Solid Edge part; units mm, degrees
sketch "Sketch1" plane through (0, 0, 0) normal (0, 0, 1) x (1, 0, 0)
  line L0 (0, 0) -> (70, 0)
  line L1 (70, 0) -> (70, 50)
  line L2 (70, 50) -> (0, 50)
  line L3 (0, 50) -> (0, 0)
extrude "Protrusion1" add sketch "Sketch1" along normal blind 5
sketch "Sketch2" plane through (0, 0, 0) normal (0, 0, 1) x (1, 0, 0)
  line L0 (25, 12.5) -> (25, 37.5)
  line L1 (25, 37.5) -> (20, 37.5)
  line L2 (20, 37.5) -> (20, 12.5)
  line L3 (20, 12.5) -> (25, 12.5)
extrude "ExtrudedProtrusion_2" add sketch "Sketch2" against normal blind 30
sketch "Sketch3" plane through (25, 25, -6.7078) normal (1, 0, 0) x (0, -1, 0)
  circle A0 centre (0, 16.5822) radius 5
extrude "ExtrudedCutout_1" cut sketch "Sketch3" against normal blind 57.348
sketch "Sketch4" plane through (35, 25, 0) normal (0, 0, -1) x (0, -1, 0)
  circle A0 centre (17, -27) radius 4
  circle A1 centre (-17, -27) radius 4
  circle A2 centre (-17, 27) radius 4
  circle A3 centre (17, 27) radius 4
extrude "ExtrudedCutout_2" cut sketch "Sketch4" against normal blind 22.6316
mirror "Mirror1" about plane through (35, 25, -6.7078) normal (1, 0, 0) of "ExtrudedProtrusion_2", "ExtrudedCutout_1"
properties material "Stainless steel"
Build history of the part. All positions in model axes, mm. A direction names the side the tool comes from. Give positions to 0.01 mm unless a question says otherwise; leave off trailing zeros. Loops run counter-clockwise (first coordinate to the right, second up) from the corner with the lowest first, then second, coordinate; pieces in that order, holes last.
Item 1: Flat gauge pins, fed straight in: pin 1 (1 mm diameter, centred on y = 27.5, z = -9, fed in from -X); pin 2 (11.5 mm diameter, centred on y = 25, z = -23.29, fed in from +X); pin 3 (2.5 mm diameter, centred on x = 21.5, z = -18.5, fed in from -Y). Where does each tip first touch, or does it go through?
Answers follow:
pin 1: stops at x = 20
pin 2: stops at x = 50
pin 3: stops at y = 12.5
Item 2: Slice it at C-C, the plane z = -27. List the corners of the cut face in (x, y), and give its area (3 significant figures).
Answers follow:
outline: (20, 12.5) - (25, 12.5) - (25, 21.65) - (20, 21.65) - close; (20, 28.35) - (25, 28.35) - (25, 37.5) - (20, 37.5) - close; (45, 12.5) - (50, 12.5) - (50, 21.65) - (45, 21.65) - close; (45, 28.35) - (50, 28.35) - (50, 37.5) - (45, 37.5) - close
area: 183 mm2
Item 3: Which spindle directions (+Z, -Z, +X, -X, +Y, -Y) get a long thin tool onto all of the face, cutting with end or side? Do faces 4 (the face through (22, 12.5, -15)), 5 (the face through (22, 25, -30)), 6 (the face through (25, 25, -15)), 7 (the face through (35, 0, 2)), 8 (the face through (20, 25, -15)). Say none if no direction does.
Answers follow:
face 4: -Z, +X, -X, -Y
face 5: -Z, +X, -X, +Y, -Y
face 6: -Z, +Y, -Y
face 7: +Z, -Z, +X, -X, -Y
face 8: -Z, -X, +Y, -Y
Item 4: Drill centre lines: line 1 (Y direction, x = 62, z = 3.45); line 2 (X direction, y = 8, z = 2); line 3 (Z direction, x = 48.85, y = 25). Where is each one in solid material? Low to high.
Answers follow:
line 1: y = 0 to 4, 12 to 38, 46 to 50
line 2: x = 0 to 4, 12 to 58, 66 to 70
line 3: z = -30 to -28.29, -18.29 to 5
Item 5: Slice it at A-A, the plane y = 8. List the corners of the cut face in (x, z).
Answers follow:
outline: (0, 0) - (4, 0) - (4, 5) - (0, 5) - close; (12, 0) - (58, 0) - (58, 5) - (12, 5) - close; (66, 0) - (70, 0) - (70, 5) - (66, 5) - close
Item 6: Pull direction Y, two halves, no side cores. Call faces 1 (the face through (50, 25, -15)), 2 (the face through (48, 37.5, -15)), 3 (the face through (47.465, 29.995, -23.07)): released by +Y, released by -Y, zero draft, split by the parting line, or undercut.
Answers follow:
face 1: zero draft
face 2: released by +Y
face 3: undercut
Item 7: Slice it at D-D, the plane y = 34. List the corners of the cut face in (x, z), and give its area (3 significant figures).
Answers follow:
outline: (0, 0) - (20, 0) - (20, -30) - (25, -30) - (25, 0) - (45, 0) - (45, -30) - (50, -30) - (50, 0) - (70, 0) - (70, 5) - (0, 5) - close
area: 650 mm2
Item 8: Slice it at B-B, the plane x = 62. List the corners of the cut face in (y, z).
Answers follow:
outline: (0, 0) - (4, 0) - (4, 5) - (0, 5) - close; (12, 0) - (38, 0) - (38, 5) - (12, 5) - close; (46, 0) - (50, 0) - (50, 5) - (46, 5) - close
